Part model, mm, in its own coordinate system. A direction names the side the tool comes from. Give positions to 0.01 mm unless a question says otherwise; leave off trailing zeros. Write each loop counter-clockwise with the first axis right and the second up, starting at its lowest first coordinate (ties: lowest second). Pieces come first, ordered by that corner, then holes.
from build123d import *

# Parameters (mm, degrees)
BOSS_EXTRUDE1_DEPTH = 50
SKETCH2_R           = 18
CUT_EXTRUDE1_DEPTH  = 50
BOSS_EXTRUDE2_DEPTH = 50
SKETCH4_W           = 40
SKETCH4_H           = 12
SKETCH4_H_2         = 13.518900255
SKETCH4_H_3         = 14.308533634
SKETCH4_H_4         = 11.829037722
CUT_EXTRUDE2_DEPTH  = 50


with BuildPart() as part:
    # Sketch1 → Boss-Extrude1 (new body)
    with BuildSketch(Plane.XY):
        with BuildLine():
            Line((-24.526421899, 99.163181947), (350.473578101, 99.163181947))
            Line((350.473578101, 99.163181947), (371.914769804, 119.776399502))
            ThreePointArc((371.914769804, 119.776399502), (379.042121684, 122.565574817), (386.05416531, 119.49802075))
            Line((386.05416531, 119.49802075), (406.845690441, 97.871359363))
            ThreePointArc((406.845690441, 97.871359363), (409.634865756, 90.744007483), (406.567311689, 83.731963857))
            Line((406.567311689, 83.731963857), (377.731763174, 56.009930349))
            Line((377.731763174, 56.009930349), (324.38122579, -54.414567916))
            Line((324.38122579, -54.414567916), (437.973578101, -220.836818053))
            Line((437.973578101, -220.836818053), (-112.026421899, -220.836818053))
            Line((-112.026421899, -220.836818053), (-12.371310843, -61.686567499))
            Line((-12.371310843, -61.686567499), (-53.371269125, 58.313432501))
            Line((-53.371269125, 58.313432501), (-86.435025525, 80.825385165))
            ThreePointArc((-86.435025525, 80.825385165), (-90.631527546, 87.226011271), (-89.072976459, 94.719312431))
            Line((-89.072976459, 94.719312431), (-72.189011961, 119.517129731))
            ThreePointArc((-72.189011961, 119.517129731), (-65.788385855, 123.713631752), (-58.295084695, 122.155080665))
            Line((-58.295084695, 122.155080665), (-24.526421899, 99.163181947))
        make_face()
        with BuildLine():
            Line((11.720938897, 49.163181947), (309.883964405, 49.163181947))
            Line((309.883964405, 49.163181947), (295.427890661, -41.493267931))
            Line((295.427890661, -41.493267931), (343.868993372, -126.082556787))
            Line((343.868993372, -126.082556787), (343.868993372, -170.836818053))
            Line((343.868993372, -170.836818053), (-26.103706827, -170.836818053))
            Line((-26.103706827, -170.836818053), (-26.103706827, -140.838487627))
            Line((-26.103706827, -140.838487627), (16.301775704, -53.067972804))
            Line((16.301775704, -53.067972804), (1.84570196, 37.588477074))
            ThreePointArc((1.84570196, 37.588477074), (4.113473855, 45.653673117), (11.720938897, 49.163181947))
        make_face(mode=Mode.SUBTRACT)
    extrude(amount=BOSS_EXTRUDE1_DEPTH)

    # Sketch2 → Cut-Extrude1 (cut)
    with BuildSketch(Plane.XY.offset(50)):
        with Locations((-57.673911362, 92.071701739)):
            Circle(SKETCH2_R)
        with Locations((373.28081392, 92.071701739)):
            Circle(SKETCH2_R)
    extrude(amount=-CUT_EXTRUDE1_DEPTH, mode=Mode.SUBTRACT)

    # Sketch3 → Boss-Extrude2 (add)
    with BuildSketch(Plane.XY.offset(50)):
        Polygon((-32.871289984, -1.686567499), (-41.412947959, 23.313432501), (-106.412947959, 23.313432501), (-106.412947959, -1.686567499), align=None)
        Polygon((-62.198866371, -141.261692776), (-46.54461658, -116.261692776), (-111.54461658, -116.261692776), (-111.54461658, -141.261692776), align=None)
        Polygon((426.934763793, 23.313432501), (361.934763793, 23.313432501), (349.856253539, -1.686567499), (426.934763793, -1.686567499), align=None)
        Polygon((431.595295067, -116.261692776), (366.595295067, -116.261692776), (383.659172075, -141.261692776), (431.595295067, -141.261692776), align=None)
    extrude(amount=-BOSS_EXTRUDE2_DEPTH)

    # Sketch4 → Cut-Extrude2 (cut)
    with BuildSketch(Plane.XY.offset(50)):
        with Locations((-86.412947959, 10.171668266)):
            Rectangle(SKETCH4_W, SKETCH4_H)
        with Locations((-91.54461658, -129.156509465)):
            Rectangle(SKETCH4_W, SKETCH4_H_2)
        with Locations((411.595295067, -128.761692776)):
            Rectangle(SKETCH4_W, SKETCH4_H_3)
        with Locations((406.934763793, 10.257149405)):
            Rectangle(SKETCH4_W, SKETCH4_H_4)
    extrude(amount=-CUT_EXTRUDE2_DEPTH, mode=Mode.SUBTRACT)


solid = part.part
1) Mould opens along X. For faces 5 (the cylindrical face through (4.035, 45.561, 24.65)), 6 (the flat face through (144, 54, 50)), 7 (the cylindrical face through (-90.61, 87.12, 24.65)) say: +X half, -X half, draft (parallel to the pull), parting line (faces both ways), or undercut.
Check result:
face 5: undercut
face 6: draft
face 7: -X half
2) Saw through at A-A (x = 287). Write the cut outline in (y, z).
Check result:
outline: (-220.84, 0) - (-170.84, 0) - (-170.84, 50) - (-220.84, 50) - close; (49.16, 0) - (99.16, 0) - (99.16, 50) - (49.16, 50) - close
3) 3-axis set-ups, long thin cutter, end or side, ignore diameter. For faces 1 (the flat face through (160, 99.163, 25)), 2 (the flat face through (9.175, -8.374, 24.65)), 3 (the flat face through (392.351, 70.065, 24.65)), 4 (the flat face through (-71.545, -129, 25)): which of +Z, -Z, +X, -X, +Y, -Y reach the whole face in a straight line?
Check result:
face 1: +Z, -Z, +Y
face 2: +Z, -Z
face 3: +Z, -Z, +X
face 4: +Z, -Z, -X
4) Drill centre lines: L1, parallel to Y at x = 54, z = 35.5; L2, parallel to Y at x = -69.5, z = 31; L3, parallel to Y at x = 0.5, z = 31.5. Where is each one in solid material? Low to high.
Check result:
L1: y = -220.84 to -170.84, 49.16 to 99.16
L2: y = -220.84 to -152.92, -141.26 to -116.26, -1.69 to 4.17, 16.17 to 23.31, 69.29 to 78.5, 105.64 to 122.19
L3: y = -220.84 to -170.84, -85.77 to 99.16
5) Saw through at C-C (z = 36). State how many separate pieces and enclosed holes the cut face has, and give its area (3 significant figures).
Check result:
separate pieces: 1
enclosed holes: 3
area: 70,100 mm2
6) Flat gauge pins, fed straight in: P1, Ø2.5, axis at y = -119.5, z = 34, coming from the +X side; P2, Ø20, axis at x = -101, z = 15, coming from the +Y side; P3, Ø6.5, axis at y = -118, z = 28.5, coming from the -X side. Where does each tip first touch, or does it go through?
Check result:
P1: stops at x = 431.6
P2: stops at y = 23.31
P3: stops at x = -111.54
7) Saw through at D-D (y = -193.5). Write the cut outline in (x, z), and give its area (3 significant figures).
Check result:
outline: (-94.91, 0) - (419.31, 0) - (419.31, 50) - (-94.91, 50) - close
area: 25,700 mm2
8) Saw through at B-B (y = -79). Write the cut outline in (x, z), and give its area (3 significant figures).
Check result:
outline: (-23.21, 0) - (3.77, 0) - (3.77, 50) - (-23.21, 50) - close; (316.91, 0) - (341.16, 0) - (341.16, 50) - (316.91, 50) - close
area: 2,560 mm2
